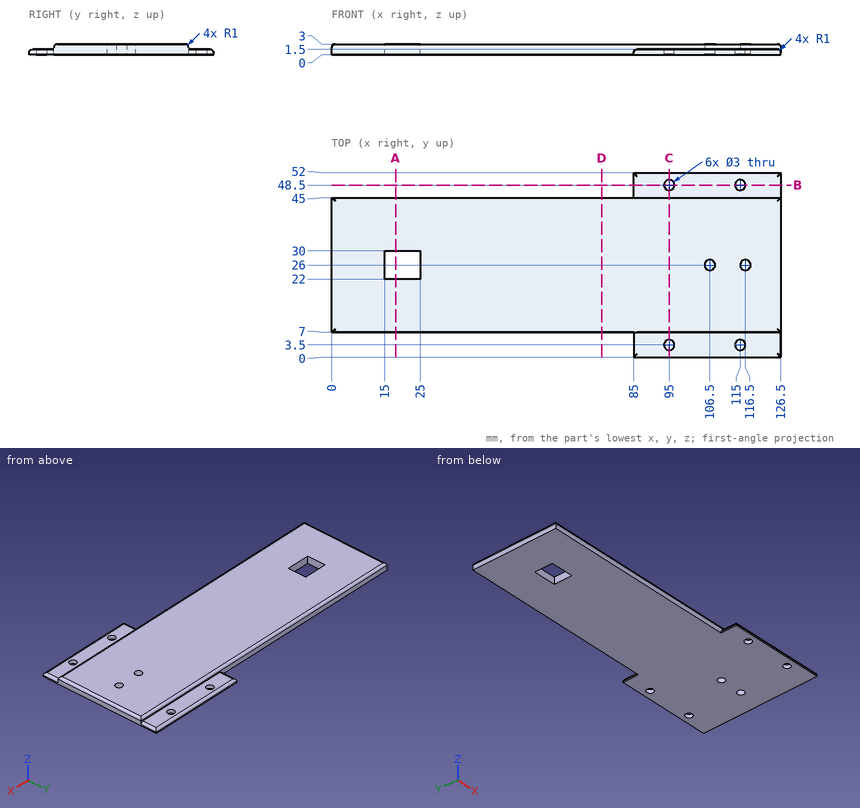
Source: three-view drawing plus pictorial views. Frame: mm from the lowest corner of the part. Round coordinates to 2 decimals unless told otherwise and drop trailing zeros. Loops run counter-clockwise (first coordinate to the right, second up) from the corner with the lowest first, then second, coordinate; pieces in that order, holes last. Notation, with made-up numbers: (0.25, 10.25) -> (19.25, 10.25) arc R16 ccw to (19.25, 19.25) -> close; hole circle Ø9 at (-19.5, -35). An arc over 180 degrees is marked (long way). Use one line per item in the form item = value.
Item 1: Cut plane B-B on y = 48.5. Output: boundary loops of the cut face in (x, z).
Evaluation:
outline = (85, 0) -> (93.5, 0) -> (93.5, 1.5) -> (86, 1.5) arc R1 ccw to (85, 0.5) -> close; (96.5, 0) -> (113.5, 0) -> (113.5, 1.5) -> (96.5, 1.5) -> close; (116.5, 0) -> (126.5, 0) -> (126.5, 0.5) arc R1 ccw to (125.5, 1.5) -> (116.5, 1.5) -> close
Item 2: Cut plane C-C on x = 95. Output: boundary loops of the cut face in (y, z), then the cut area to 3 significant figures.
Evaluation:
outline = (0, 0) -> (2, 0) -> (2, 1.5) -> (1, 1.5) arc R1 ccw to (0, 0.5) -> close; (5, 0) -> (47, 0) -> (47, 1.5) -> (45, 1.5) -> (45, 2) arc R1 ccw to (44, 3) -> (8, 3) arc R1 ccw to (7, 2) -> (7, 1.5) -> (5, 1.5) -> close; (50, 0) -> (52, 0) -> (52, 0.5) arc R1 ccw to (51, 1.5) -> (50, 1.5) -> close
area = 125 mm2
Item 3: Contact query for flat-ended pins moving along their axis: pin 1 Ø2.5 at (x, y) = (95, 3.5) entering from +Z; pin 2 Ø0.9 at (x, z) = (20, 1) entering from +Y; pin 3 Ø0.6 at (x, z) = (84.5, 1.5) entering from -Y; pin 4 Ø4 at (x, y) = (115, 48.5) entering from +Z. Output: stop coordinate, or through.
Evaluation:
pin_1 = through
pin_2 = 45
pin_3 = 7
pin_4 = 1.5
Item 4: Cut plane A-A on x = 18. Output: boundary loops of the cut face in (y, z), then the cut area to 3 significant figures.
Evaluation:
outline = (7, 0) -> (22, 0) -> (22, 3) -> (8, 3) arc R1 ccw to (7, 2) -> close; (30, 0) -> (45, 0) -> (45, 2) arc R1 ccw to (44, 3) -> (30, 3) -> close
area = 89.6 mm2
Item 5: Material intervals for probe 1 along X at (y, z) = (27, 2.3); probe 2 along Y at (x, z) = (23.5, 0.8); probe 3 along X at (y, z) = (36, 2.05), sorted ascending.
Evaluation:
probe_1 = 0.05 to 15, 25 to 105.38, 107.62 to 115.38, 117.62 to 126.45
probe_2 = 7 to 22, 30 to 45
probe_3 = 0 to 126.5
Item 6: Cut plane D-D on x = 76. Output: boundary loops of the cut face in (y, z), then the cut area to 3 significant figures.
Evaluation:
outline = (7, 0) -> (45, 0) -> (45, 2) arc R1 ccw to (44, 3) -> (8, 3) arc R1 ccw to (7, 2) -> close
area = 114 mm2
